```python
from build123d import *

# Parameters (mm, degrees)
SKETCH1_W           = 5
SKETCH1_H           = 5
BOSS_EXTRUDE1_DEPTH = 10
BOSS_EXTRUDE2_DEPTH = 1.5


with BuildPart() as part:
    # Sketch1 → Boss-Extrude1 (new, symmetric)
    with BuildSketch(Plane.XY):
        Rectangle(SKETCH1_W, SKETCH1_H)
    extrude(amount=BOSS_EXTRUDE1_DEPTH, both=True)

    # Sketch2 → Boss-Extrude2 (add, symmetric)
    with BuildSketch(Plane.XY):
        with BuildLine():
            Line((0, 0.25), (-2.5, 0.25))
            ThreePointArc((-2.5, 0.25), (-7.5, 5.25), (-2.5, 10.25))
            Line((-2.5, 10.25), (0, 10.25))
            Line((0, 10.25), (0, 10.75))
            Line((0, 10.75), (-2.5, 10.75))
            ThreePointArc((-2.5, 10.75), (-8, 5.25), (-2.5, -0.25))
            Line((-2.5, -0.25), (0, -0.25))
            Line((0, -0.25), (0, 0.25))
        make_face()
    boss_extrude2 = extrude(amount=BOSS_EXTRUDE2_DEPTH, both=True)

    # Mirror1: Boss-Extrude2 across plane
    add(boss_extrude2.mirror(Plane(origin=(0, 0, 0), x_dir=(0, 0, 1), z_dir=(1, 0, 0))))

    # Sketch3 → Revolve3 (revolve)
    with BuildSketch(Plane.XY):
        with BuildLine():
            Line((0, 10.5), (0, 20.5))
            ThreePointArc((0, 20.5), (-5, 15.5), (0, 10.5))
        make_face()
    revolve(axis=Axis((0, 0, 0), (0, 1, 0)))


solid = part.part
```
Here's how the part is built. I have some questions about the finished solid (model axes, mm). A direction names the side the tool comes from. Coordinates: 2 decimals unless noted, no trailing zeros. Loops run counter-clockwise (first coordinate to the right, second up) from the corner with the lowest first, then second, coordinate; pieces in that order, holes last. Notation, with made-up numbers: (-21, 15) - (-1, 15) arc R21 cw to (-1, 50) - close; hole circle Ø3 at (23, 18). An arc over 180 degrees is marked (long way). Return JSON: item names as keys, results as strings. Group by question number.
Item 1: If we section it at C-C on y = 1: Write out the boundary of the cut face in (x, z), and give its area (3 significant figures).
Item 2: On a 3-axis mill with a long thin cutter (end or side, diameter ignored), from which of +Z, -Z, +X, -X, +Y, -Y can I reach the whole of each face in a straight line? I mean faces 1 (the face through (8, 5.37, 0.02)), 2 (the face through (7.5, 5.14, 0.02)). Say none if no direction works.
Item 3: I need wall thicknesses on line 1 (X direction, y = 2, z = 0); line 2 (Y direction, x = -2.75, z = 1.25); line 3 (Z direction, x = -7, y = 2.25). Which ranges of each line are inside material? Lowest first, please. Write a range as from..to.
Item 4: If we section it at A-A on y = 5.25: Write out the boundary of the cut face in (x, z).
Item 5: Will these pins go through, and if not, where does the flat tip stop? P1, Ø2.5, axis at y = -0.5, z = 1.5, coming from the +X side; P2, Ø0.6, axis at x = -1, z = -0.5, coming from the +Y side; P3, Ø2.5, axis at y = 0.5, z = -2, coming from the -X side.
Item 6: If we section it at D-D on z = -1: Write out the boundary of the cut face in (x, y).
Item 7: If we section it at B-B on x = 7: Write out the boundary of the cut face in (y, z), and give its area (3 significant figures).
Item 8: We'd pull the mould along Y, two halves only. Please class faces 3 (the face through (0, 0, -10)), 4 (the face through (0, 2.5, 0)), 5 (the face through (0, -2.5, 0)): +Y half, -Y half, draft (parallel to the pull), parting line (faces both ways), or undercut.
Calculated:
{
 "1": {"outline": "(-5.99, -1.5) - (-5.13, -1.5) - (-5.13, 1.5) - (-5.99, 1.5) - close; (-2.5, -10) - (2.5, -10) - (2.5, 10) - (-2.5, 10) - close; (5.13, -1.5) - (5.99, -1.5) - (5.99, 1.5) - (5.13, 1.5) - close", "area": "105 mm^2"},
 "2": {"face 1": "+Z, -Z, +X", "face 2": "+Z, -Z"},
 "3": {"line 1": "x = -6.94..-6.3, -2.5..2.5, 6.3..6.94", "line 2": "y = -0.24..0.26, 10.24..10.74, 11.52..19.48", "line 3": "z = -1.5..1.5"},
 "4": {"outline": "(-8, -1.5) - (-7.5, -1.5) - (-7.5, 1.5) - (-8, 1.5) - close; (7.5, -1.5) - (8, -1.5) - (8, 1.5) - (7.5, 1.5) - close"},
 "5": {"P1": "stops at x = 5.66", "P2": "stops at y = 20.43", "P3": "stops at x = -6.65"},
 "6": {"outline": "(-2.5, -2.5) - (2.5, -2.5) - (2.5, -0.25) arc R5.5 ccw to (2.5, 10.75) - (1.2, 10.75) arc R4.9 ccw (long way) to (-1.2, 10.75) - (-2.5, 10.75) arc R5.5 ccw to (-2.5, -0.25) - close; hole (-2.5, 0.25) - (-2.5, 2.5) - (2.5, 2.5) - (2.5, 0.25) arc R5 ccw to (2.5, 10.25) - (-2.5, 10.25) arc R5 ccw to start"},
 "7": {"outline": "(2.09, -1.5) - (3.07, -1.5) - (3.07, 1.5) - (2.09, 1.5) - close; (7.43, -1.5) - (8.41, -1.5) - (8.41, 1.5) - (7.43, 1.5) - close", "area": "5.90 mm^2"},
 "8": {"face 3": "draft", "face 4": "undercut", "face 5": "-Y half"}
}
